Autodesk Inventor part; units mm, degrees
ref_plane "YZ Plane" through (0, 0, 0) normal (1, 0, 0) x (0, 1, 0)
ref_plane "XZ Plane" through (0, 0, 0) normal (0, 1, 0) x (-1, 0, 0)
ref_plane "XY Plane" through (0, 0, 0) normal (0, 0, 1) x (1, 0, 0)
sketch "Sketch1" plane through (0, 0, 0) normal (0, 0, 1) x (1, 0, 0)
  line L0 (90, 0) -> (90, -3)
  line L1 (60, -3) -> (60, 0)
  line L2 (0, 60) -> (0, 45)
  line L3 (3, 45) -> (3, 15)
  line L4 (0, 45) -> (3, 45)
  line L5 (3, 15) -> (0, 15)
  line L6 (0, 15) -> (0, 0)
  line L7 (90, -3) -> (60, -3)
  line L8 (90, 0) -> (150, 0)
  line L9 (150, 60) -> (0, 60)
  line L10 (150, 15) -> (147, 15)
  line L11 (147, 15) -> (147, 45)
  line L12 (147, 45) -> (150, 45)
  line L13 (150, 0) -> (150, 15)
  line L14 (150, 45) -> (150, 60)
  line L15 (35.3315, 0) -> (35.3315, 15)
  line L16 (35.3315, 15) -> (20.3315, 15)
  line L17 (20.3315, 15) -> (20.3315, 0)
  line L18 (0, 0) -> (20.3315, 0)
  line L19 (35.3315, 0) -> (60, 0)
  dimension "d10" = 150
  dimension "d11" = 60
  dimension "d12" = 3
  dimension "d13" = 15
  dimension "d14" = 3
  dimension "d15" = 30
  dimension "d16" = 30
  dimension "d17" = 3
  dimension "d18" = 3
  dimension "d19" = 15
extrude "Extrusion1" add sketch "Sketch1" along normal blind 3
properties part number "atas"
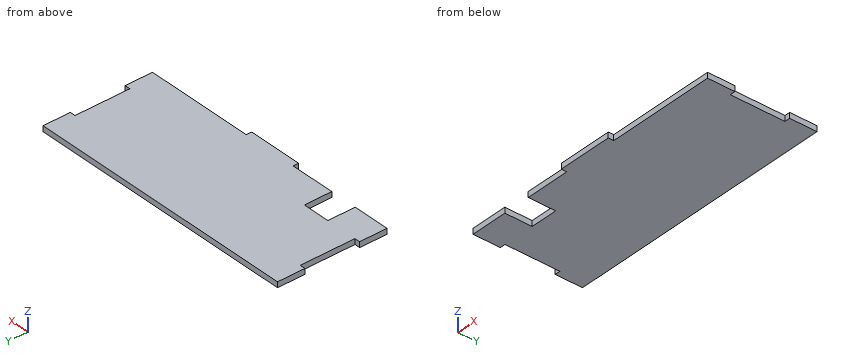
The listing builds one solid part. Answer for the finished solid, in the listing's coordinates (mm). Round coordinates to 2 decimals unless told otherwise and drop trailing zeros. Write each loop counter-clockwise with the first axis right and the second up, starting at its lowest first coordinate (ties: lowest second). Pieces come first, ordered by that corner, then holes. Notation, with made-up numbers: (8.25, 50.5) - (32.25, 50.5) arc R27 ccw to (32.25, 82.5) - close; hole circle Ø2 at (32.25, 14.25). An arc over 180 degrees is marked (long way). Use a Markdown table: item, result. Add a question column.
1. The part is cut by section B-B (z = 1.2). Write down the section's boundary in (x, y), and give its area (4 significant figures).
2. The part is cut by section A-A (y = 13). Write down the section's boundary in (x, z).
3. The part is cut by section C-C (y = 23). Write down the section's boundary in (x, z).
4. Consider line 1 (X direction, y = 6, z = 1); line 2 (X direction, y = 29, z = 0.2); line 3 (Y direction, x = 107, z = 1.75). Determine where each line is inside the solid, lowest interval first.
5. The part is cut by section D-D (x = 45). Write down the section's boundary in (y, z), and give its area (3 significant figures).
Reported:
| question | item | result |
|---|---|---|
| 1 | outline | (0, 0) - (20.33, 0) - (20.33, 15) - (35.33, 15) - (35.33, 0) - (60, 0) - (60, -3) - (90, -3) - (90, 0) - (150, 0) - (150, 15) - (147, 15) - (147, 45) - (150, 45) - (150, 60) - (0, 60) - (0, 45) - (3, 45) - (3, 15) - (0, 15) - close |
| 1 | area | 8,685 mm^2 |
| 2 | outline | (0, 0) - (20.33, 0) - (20.33, 3) - (0, 3) - close; (35.33, 0) - (150, 0) - (150, 3) - (35.33, 3) - close |
| 3 | outline | (3, 0) - (147, 0) - (147, 3) - (3, 3) - close |
| 4 | line 1 | 0 to 20.33, 35.33 to 150 |
| 4 | line 2 | 3 to 147 |
| 4 | line 3 | 0 to 60 |
| 5 | outline | (0, 0) - (60, 0) - (60, 3) - (0, 3) - close |
| 5 | area | 180 mm^2 |
